Job drawing, mm, ordinate dimensions from the low corner. One solid piece. A direction names the side the tool comes from. Round coordinates to 2 decimals unless told otherwise and drop trailing zeros. Write each loop counter-clockwise with the first axis right and the second up, starting at its lowest first coordinate (ties: lowest second). Pieces come first, ordered by that corner, then holes. Notation, with made-up numbers: (-28.75, 39.25) -> (27.25, 39.25) arc R20 ccw to (27.25, 46.25) -> close; hole circle Ø7 at (80, -20). An arc over 180 degrees is marked (long way). Use CSV: the item, a comma, the result in double quotes. Start each with the question number.
(1) Probe line 1 (Y direction, x = 9.5, z = 3.65) (1 decimal); line 2 (X direction, y = 13, z = 0.35). List the from-to ranges inside material, lowest first. Write a range as [from, to].
(2) Saw through at A-A (y = 11). Give the cut face in (x, z).
(3) Which spindle directions (+Z, -Z, +X, -X, +Y, -Y) get a long thin tool onto all of the face, cutting with end or side? Do the marked faces 1, 2 and 3. Say none if no direction does.
(4) Two-plate mould, pull along Y, no slides. Class the marked faces 4, 5 and 6: released by +Y, released by -Y, zero draft, split by the parting line, or undercut.
(5) Saw through at B-B (z = 0.55). Give the cut face in (x, y).
(6) Drop flat-ended pins along their axis: pin 1 (4 mm diameter, centred on x = 10, y = 13, fed in from -Z); pin 2 (3 mm diameter, centred on x = 3, z = 1.5, fed in from -Y) (1 decimal); pin 3 (1.6 mm diameter, centred on x = 19, y = 11, fed in from +Z); pin 4 (1.5 mm diameter, centred on y = 10, z = 3.5, fed in from -X). Give the stop position or say it passes through.
(7) Saw through at C-C (x = 19). Give the cut face in (y, z).
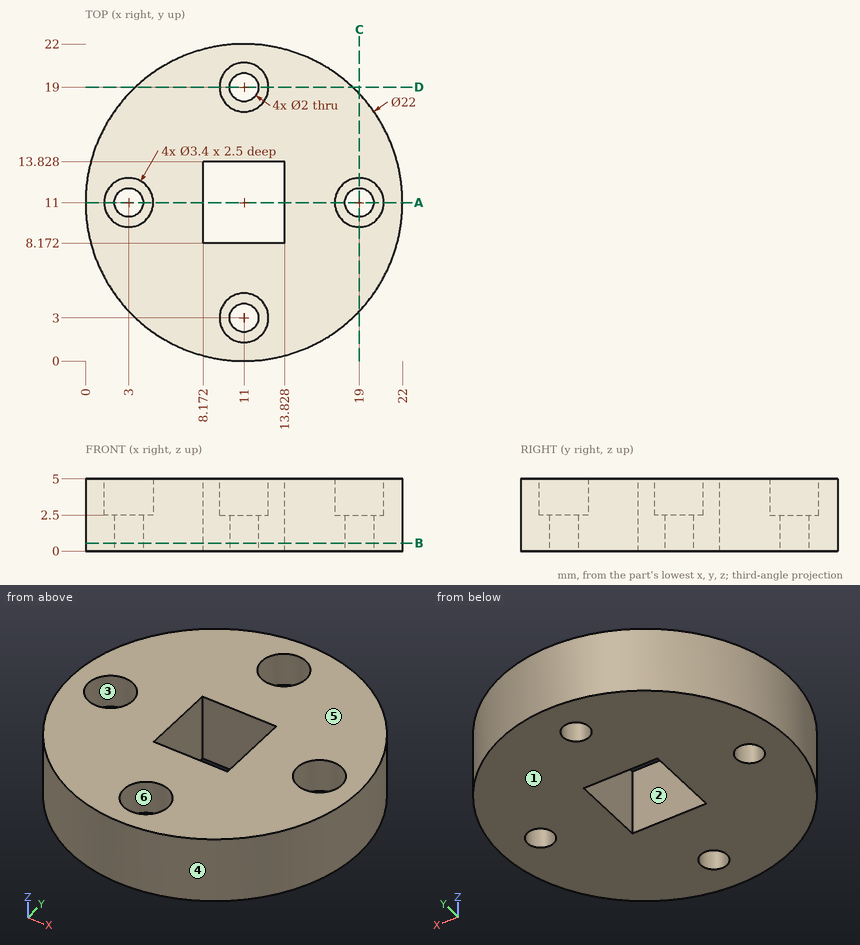
Answers:
1,line 1,"y = [0.1, 2.2], [3.8, 8.2], [13.8, 18.2], [19.8, 21.9]"
1,line 2,"x = [0.18, 8.17], [13.83, 21.82]"
2,outline,"(0, 0) -> (2, 0) -> (2, 2.5) -> (1.3, 2.5) -> (1.3, 5) -> (0, 5) -> close; (4, 0) -> (8.17, 0) -> (8.17, 5) -> (4.7, 5) -> (4.7, 2.5) -> (4, 2.5) -> close; (13.83, 0) -> (18, 0) -> (18, 2.5) -> (17.3, 2.5) -> (17.3, 5) -> (13.83, 5) -> close; (20, 0) -> (22, 0) -> (22, 5) -> (20.7, 5) -> (20.7, 2.5) -> (20, 2.5) -> close"
3,face 1,"-Z, +X, -X, +Y, -Y"
3,face 2,"+Z, -Z"
3,face 3,"+Z"
4,face 4,"split by the parting line"
4,face 5,"zero draft"
4,face 6,"undercut"
5,outline,"circle Ø22 at (11, 11); hole circle Ø2 at (3, 11); hole (8.17, 8.17) -> (13.83, 8.17) -> (13.83, 13.83) -> (8.17, 13.83) -> close; hole circle Ø2 at (11, 3); hole circle Ø2 at (11, 19); hole circle Ø2 at (19, 11)"
6,pin 1,"stops at z = 0"
6,pin 2,"stops at y = 2.1"
6,pin 3,"passes through"
6,pin 4,"stops at x = 0"
7,outline,"(3.45, 0) -> (10, 0) -> (10, 2.5) -> (9.3, 2.5) -> (9.3, 5) -> (3.45, 5) -> close; (12, 0) -> (18.55, 0) -> (18.55, 5) -> (12.7, 5) -> (12.7, 2.5) -> (12, 2.5) -> close"
